Work out the finished part from the listing and answer in its coordinate system (mm). A direction names the side the tool comes from. Coordinates: 2 decimals unless noted, no trailing zeros. Order: outer loops, then holes, each group sorted by start corner. A loop starts at its lowest first (then second) coordinate and runs counter-clockwise, first axis right, second up. Notation, with made-up numbers: (77.25, -27.75) -> (122.25, -27.75) arc R17 cw to (122.25, -3.75) -> close; hole circle Ø2 at (79.5, -9). An arc over 180 degrees is marked (long way). Use one line per item in the form item = value.
from build123d import *

# Parameters (mm, degrees)
F1_DEPTH     = 2
F2_R         = 3
F0_W         = 55
F0_H         = 20
F0_W_2       = 38
F0_H_2       = 15
F3_DEPTH     = 2
F4_R         = 3
F5_T1_DEPTH  = 38
F5_T3_DEPTH  = 15
F5_T9_DEPTH  = 44.1720391711
F5_T13_DEPTH = 21.1720391711
F5_T20_DEPTH = 44.1720391711
F5_T24_DEPTH = 21.1720391711
F5_T31_DEPTH = 21.1720391711
F5_T35_DEPTH = 44.1720391711
F5_T42_DEPTH = 44.1720391711
F5_T46_DEPTH = 21.1720391711
F8_START     = -23.1
F7_W         = 7.2
F7_H         = 3.4
F8_DEPTH     = 9.4
F9_START     = -23.1
F7_H_2       = 2.4
F9_DEPTH     = 11.8
F10_SIZE     = 2
F11_T4_DEPTH = 17.4867319519
F11_T9_DEPTH = 17.4867319519


# Not quite as in the source:
# - a fillet or chamfer that OpenCascade refuses, or shapes differently, is made with other operations: its cross-section is extruded or revolved along the edge and cut away or added
# - a feature names something its author has since deleted; it is built from what else it names


with BuildPart() as f1:
    # F0 (on Top) → F1 (new body)
    with BuildSketch(Plane.XY):
        with BuildLine():
            Line((42.8, 7.5), (46.1, 7.5))
            Line((46.1, 7.5), (46.1, 21.5))
            Line((46.1, 21.5), (-8.9, 21.5))
            Line((-8.9, 21.5), (-8.9, 41.5))
            Line((-8.9, 41.5), (-30.9, 41.5))
            Line((-30.9, 41.5), (-30.9, -33.5))
            Line((-30.9, -33.5), (46.1, -33.5))
            Line((46.1, -33.5), (46.1, -7.5))
            Line((46.1, -7.5), (42.8, -7.5))
            ThreePointArc((42.8, -7.5), (35.3, 0), (42.8, 7.5))
        make_face()
    extrude(amount=-F1_DEPTH)

    # F2
    f2_edges = [f1.edges().sort_by_distance(p)[0] for p in [
        (46.1, -33.5, -1),
        (-30.9, -33.5, -1),
        (-30.9, 41.5, -1),
    ]]
    fillet(f2_edges, radius=F2_R)

    # F0 (on Top) → F3 (join)
    with BuildSketch(Plane.XY):
        with Locations((18.6, 31.5)):
            Rectangle(F0_W, F0_H)
        with Locations((19, 32.5)):
            Rectangle(F0_W_2, F0_H_2, mode=Mode.SUBTRACT)
        with BuildLine():
            Line((42.8, 7.5), (46.1, 7.5))
            Line((46.1, 7.5), (46.1, 21.5))
            Line((46.1, 21.5), (-8.9, 21.5))
            Line((-8.9, 21.5), (-8.9, 41.5))
            Line((-8.9, 41.5), (-30.9, 41.5))
            Line((-30.9, 41.5), (-30.9, -33.5))
            Line((-30.9, -33.5), (46.1, -33.5))
            Line((46.1, -33.5), (46.1, -7.5))
            Line((46.1, -7.5), (42.8, -7.5))
            ThreePointArc((42.8, -7.5), (35.3, 0), (42.8, 7.5))
        make_face()
        with BuildLine():
            Line((42.8, 1.5), (42.8, 7.5))
            ThreePointArc((42.8, 7.5), (35.3, 0), (42.8, -7.5))
            Line((42.8, -7.5), (42.8, -1.5))
            ThreePointArc((42.8, -1.5), (41.3, 0), (42.8, 1.5))
        make_face()
        with BuildLine():
            Line((46.1, -6.7349832962), (46.1, 6.7349832962))
            ThreePointArc((46.1, 6.7349832962), (44.4937569599, 7.3062430401), (42.8, 7.5))
            Line((42.8, 7.5), (42.8, 1.5))
            ThreePointArc((42.8, 1.5), (43.8606601718, 1.0606601718), (44.3, 0))
            ThreePointArc((44.3, 0), (43.8606601718, -1.0606601718), (42.8, -1.5))
            Line((42.8, -1.5), (42.8, -7.5))
            ThreePointArc((42.8, -7.5), (44.4937569599, -7.3062430401), (46.1, -6.7349832962))
        make_face()
        with BuildLine():
            Line((46.1, -7.5), (46.1, -6.7349832962))
            ThreePointArc((46.1, -6.7349832962), (44.4937569599, -7.3062430401), (42.8, -7.5))
            Line((42.8, -7.5), (46.1, -7.5))
        make_face()
        with BuildLine():
            Line((50, 45), (-34.8, 45))
            Line((-34.8, 45), (-34.8, -37))
            Line((-34.8, -37), (50, -37))
            Line((50, -37), (50, -2.1))
            ThreePointArc((50, -2.1), (48.538751392, -4.8287402561), (46.1, -6.7349832962))
            Line((46.1, -6.7349832962), (46.1, -7.5))
            Line((46.1, -7.5), (46.1, -33.5))
            Line((46.1, -33.5), (-30.9, -33.5))
            Line((-30.9, -33.5), (-30.9, 41.5))
            Line((-30.9, 41.5), (-8.9, 41.5))
            Line((-8.9, 41.5), (46.1, 41.5))
            Line((46.1, 41.5), (46.1, 21.5))
            Line((46.1, 21.5), (46.1, 7.5))
            Line((46.1, 7.5), (46.1, 6.7349832962))
            ThreePointArc((46.1, 6.7349832962), (48.538751392, 4.8287402561), (50, 2.1))
            Line((50, 2.1), (50, 45))
        make_face()
        with BuildLine():
            Line((50, -2.1), (50, 2.1))
            ThreePointArc((50, 2.1), (48.538751392, 4.8287402561), (46.1, 6.7349832962))
            Line((46.1, 6.7349832962), (46.1, -6.7349832962))
            ThreePointArc((46.1, -6.7349832962), (48.538751392, -4.8287402561), (50, -2.1))
        make_face()
        with BuildLine():
            ThreePointArc((42.8, 7.5), (44.4937569599, 7.3062430401), (46.1, 6.7349832962))
            Line((46.1, 6.7349832962), (46.1, 7.5))
            Line((46.1, 7.5), (42.8, 7.5))
        make_face()
    extrude(amount=F3_DEPTH)

    # F4
    f4_edges = [f1.edges().sort_by_distance(p)[0] for p in [
        (50, -37, 1),
        (-34.8, -37, 1),
        (-34.8, 45, 1),
        (50, 45, 1),
    ]]
    fillet(f4_edges, radius=F4_R)

    # F5: chamfer of 2.4 on 4 edges, made by hand

    # F5_s2 → F5_t1 (cut)
    with BuildSketch(Plane.YZ):
        Polygon((42.4, 2), (40, -0.4), (40, 2), align=None)
        Polygon((22.6, 2), (25, -0.4), (25, 2), align=None)
    extrude(amount=F5_T1_DEPTH, mode=Mode.SUBTRACT)

    # F5_s4 → F5_t3 (cut)
    with BuildSketch(Plane.XZ.offset(-40)):
        Polygon((40.4, 2), (38, -0.4), (38, 2), align=None)
        Polygon((-2.4, 2), (0, -0.4), (0, 2), align=None)
    extrude(amount=F5_T3_DEPTH, mode=Mode.SUBTRACT)


with BuildPart() as f5_tool7:
    # F5_s8 → F5_t9 (new body)
    with BuildSketch(Plane.YZ.offset(-6.1720391711)):
        Polygon((42.4, 2), (40, -0.4), (40, 2), align=None)
    extrude(amount=F5_T9_DEPTH)

    split(bisect_by=Plane.YZ, keep=Keep.BOTTOM)


with BuildPart() as f5_tool11:
    # F5_s12 → F5_t13 (new body)
    with BuildSketch(Plane.XZ.offset(-25)):
        Polygon((-2.4, 2), (0, -0.4), (0, 2), align=None)
    extrude(amount=-F5_T13_DEPTH)

    split(bisect_by=Plane.XZ.offset(-40), keep=Keep.BOTTOM)


with BuildPart() as f5_tool7_1:
    add(f5_tool7.part)

    # F5_t15: intersect F5_tool11
    add(f5_tool11.part, mode=Mode.INTERSECT)


with BuildPart() as f1_1:
    add(f1.part)

    # F5_t5: cut F5_tool7
    add(f5_tool7_1.part, mode=Mode.SUBTRACT)


with BuildPart() as f5_tool18:
    # F5_s19 → F5_t20 (new body)
    with BuildSketch(Plane.YZ):
        Polygon((42.4, 2), (40, -0.4), (40, 2), align=None)
    extrude(amount=F5_T20_DEPTH)

    split(bisect_by=Plane.YZ.offset(38), keep=Keep.TOP)


with BuildPart() as f5_tool22:
    # F5_s23 → F5_t24 (new body)
    with BuildSketch(Plane.XZ.offset(-46.1720391711)):
        Polygon((40.4, 2), (38, -0.4), (38, 2), align=None)
    extrude(amount=F5_T24_DEPTH)

    split(bisect_by=Plane.XZ.offset(-40), keep=Keep.BOTTOM)


with BuildPart() as f5_tool18_1:
    add(f5_tool18.part)

    # F5_t26: intersect F5_tool22
    add(f5_tool22.part, mode=Mode.INTERSECT)


with BuildPart() as f1_2:
    add(f1_1.part)

    # F5_t16: cut F5_tool18
    add(f5_tool18_1.part, mode=Mode.SUBTRACT)


with BuildPart() as f5_tool29:
    # F5_s30 → F5_t31 (new body)
    with BuildSketch(Plane.XZ.offset(-40)):
        Polygon((40.4, 2), (38, -0.4), (38, 2), align=None)
    extrude(amount=F5_T31_DEPTH)

    split(bisect_by=Plane.XZ.offset(-25), keep=Keep.TOP)


with BuildPart() as f5_tool33:
    # F5_s34 → F5_t35 (new body)
    with BuildSketch(Plane.YZ.offset(44.1720391711)):
        Polygon((22.6, 2), (25, -0.4), (25, 2), align=None)
    extrude(amount=-F5_T35_DEPTH)

    split(bisect_by=Plane.YZ.offset(38), keep=Keep.TOP)


with BuildPart() as f5_tool29_1:
    add(f5_tool29.part)

    # F5_t37: intersect F5_tool33
    add(f5_tool33.part, mode=Mode.INTERSECT)


with BuildPart() as f1_3:
    add(f1_2.part)

    # F5_t27: cut F5_tool29
    add(f5_tool29_1.part, mode=Mode.SUBTRACT)


with BuildPart() as f5_tool40:
    # F5_s41 → F5_t42 (new body)
    with BuildSketch(Plane.YZ.offset(38)):
        Polygon((22.6, 2), (25, -0.4), (25, 2), align=None)
    extrude(amount=-F5_T42_DEPTH)

    split(bisect_by=Plane.YZ, keep=Keep.BOTTOM)


with BuildPart() as f5_tool44:
    # F5_s45 → F5_t46 (new body)
    with BuildSketch(Plane.XZ.offset(-18.8279608289)):
        Polygon((-2.4, 2), (0, -0.4), (0, 2), align=None)
    extrude(amount=-F5_T46_DEPTH)

    split(bisect_by=Plane.XZ.offset(-25), keep=Keep.TOP)


with BuildPart() as f5_tool40_1:
    add(f5_tool40.part)

    # F5_t48: intersect F5_tool44
    add(f5_tool44.part, mode=Mode.INTERSECT)


with BuildPart() as f1_4:
    add(f1_3.part)

    # F5_t38: cut F5_tool40
    add(f5_tool40_1.part, mode=Mode.SUBTRACT)

    # F6: chamfer of 3 on 1 edges, made by hand

    # F6_s1 → F6_t2 (revolve, cut)
    with BuildSketch(Plane.YZ.offset(42.8)):
        Polygon((4.5, 2), (1.5, -1), (1.5, 2), align=None)
    revolve(axis=Axis((42.8, 0, 2), (0, 0, -1)), mode=Mode.SUBTRACT)

    # F7 (on Right) → F8 (join)
    with BuildSketch(Plane.YZ.offset(F8_START)):
        with Locations((28.0882296383, -3.7)):
            Rectangle(F7_W, F7_H)
        with Locations((-20.1117703617, -3.7)):
            Rectangle(F7_W, F7_H)
    extrude(amount=-F8_DEPTH)

    # F7 (on Right) → F9 (join)
    with BuildSketch(Plane.YZ.offset(F9_START)):
        with Locations((28.0882296383, -6.6)):
            Rectangle(F7_W, F7_H_2)
        with Locations((-20.1117703617, -6.6)):
            Rectangle(F7_W, F7_H_2)
    extrude(amount=-F9_DEPTH)

    # F10
    f10_edges = [f1_4.edges().sort_by_distance(p)[0] for p in [
        (-23.1, -20.11177, -7.8),
        (-23.1, 28.08823, -7.8),
    ]]
    chamfer(f10_edges, length=F10_SIZE)

    # F11: chamfer of 2 on 2 edges, made by hand


with BuildPart() as f11_tool2:
    # F11_s3 → F11_t4 (new body)
    with BuildSketch(Plane.XZ.offset(11.3684043857)):
        Polygon((-30.5, -2), (-32.5, -4), (-32.5, -2), align=None)
    extrude(amount=F11_T4_DEPTH)

    split(bisect_by=Plane.YZ.offset(-30.9), keep=Keep.BOTTOM)


with BuildPart() as f1_5:
    add(f1_4.part)

    # F11_t1: cut F11_tool2
    add(f11_tool2.part, mode=Mode.SUBTRACT)


with BuildPart() as f11_tool7:
    # F11_s8 → F11_t9 (new body)
    with BuildSketch(Plane.XZ.offset(-36.8315956143)):
        Polygon((-30.5, -2), (-32.5, -4), (-32.5, -2), align=None)
    extrude(amount=F11_T9_DEPTH)

    split(bisect_by=Plane.YZ.offset(-30.9), keep=Keep.BOTTOM)


with BuildPart() as f1_6:
    add(f1_5.part)

    # F11_t6: cut F11_tool7
    add(f11_tool7.part, mode=Mode.SUBTRACT)


solid = f1_6.part
(1) Which of the six approach directions +Z, -Z, +X, -X, +Y, -Y give full straight-line access (tool end or side, diameter ignored) to faces 1 (the flat face through (7, -33.5, -1)), 2 (the flat face through (-34.8, 5, 1)), 3 (the flat face through (-34, 28, -5.4)), 4 (the flat face through (-23.1, -20, -4))?
Data:
face_1 = -Z, +X, -X, -Y
face_2 = +Z, -X, +Y, -Y
face_3 = -X, +Y, -Y
face_4 = -Z, +X, +Y, -Y
(2) Section B-B on y = 27 is taken. Write down the section's boundary in (x, z).
Data:
outline = (-34.9, -7.8) -> (-25.1, -7.8) -> (-23.1, -5.8) -> (-23.1, -2) -> (-8.9, -2) -> (-8.9, 0) -> (-0.4, 0) -> (-2.4, 2) -> (-34.8, 2) -> (-34.8, 0) -> (-30.9, 0) -> (-30.9, -2.4) -> (-32.5, -4) -> (-32.5, -5.4) -> (-34.9, -5.4) -> close; (38.4, 0) -> (50, 0) -> (50, 2) -> (40.4, 2) -> close
(3) Each of these flat-tipped pins is pushed along its axis until it touches: P1, Ø1.6, axis at x = 19.5, z = -1, coming from the +Y side; P2, Ø1.7, axis at x = -28, z = -5.5, coming from the +Y side; P3, Ø1.5, axis at y = -22.5, z = -2, coming from the +X side. Where does it stop, or does it pass through?
Data:
P1 = 21.5
P2 = 31.69
P3 = 46.1
(4) Section D-D on y = 37.5 is taken. Write down the section's boundary in (x, z), plus the area to 3 significant figures.
Data:
outline = (-34.8, 0) -> (-30.9, 0) -> (-30.9, -2) -> (-8.9, -2) -> (-8.9, 0) -> (-0.4, 0) -> (-2.4, 2) -> (-34.8, 2) -> close; (38.4, 0) -> (50, 0) -> (50, 2) -> (40.4, 2) -> close
area = 132 mm²
(5) Section C-C on x = -13 is taken. Write down the section's boundary in (y, z).
Data:
outline = (-37, 0) -> (-33.5, 0) -> (-33.5, -2) -> (41.5, -2) -> (41.5, 0) -> (45, 0) -> (45, 2) -> (-37, 2) -> close
(6) The mould has two halves that part along Y. Classify faces 5 (the flat face through (-29, -16.512, -5)), 6 (the flat face through (19, 21.5, -1)), 7 (the cylindrical face through (-33.9, -36.14, 1.01)): released by +Y, released by -Y, zero draft, split by the parting line, or undercut.
Data:
face_5 = undercut
face_6 = released by +Y
face_7 = released by -Y
(7) Straight lines are drawn through the part: line 1 along Y through (x, z) = (-29, -7.5); line 2 along Z through (x, y) = (-20, 15); line 3 along X through (y, z) = (19, 1.5). For each, find the intervals that lie inside material, in ascending order.
Data:
line_1 = -23.71 to -16.51, 24.49 to 31.69
line_2 = -2 to 2
line_3 = -34.8 to 50
(8) Section A-A on x = 18 is taken. Write down the section's boundary in (y, z), plus the area to 3 significant figures.
Data:
outline = (-37, 0) -> (-33.5, 0) -> (-33.5, -2) -> (21.5, -2) -> (21.5, 0) -> (24.6, 0) -> (22.6, 2) -> (-37, 2) -> close; (40.4, 0) -> (45, 0) -> (45, 2) -> (42.4, 2) -> close
area = 238 mm²
